Could you check a few things on this model? Use its own coordinates, in mm. A direction names the side the tool comes from. Round coordinates to 2 decimals unless told otherwise and drop trailing zeros. Order: outer loops, then holes, each group sorted by start corner. A loop starts at its lowest first (then second) coordinate and runs counter-clockwise, first axis right, second up.
```python
from build123d import *

# Parameters (mm, degrees)
RESSALTO_EXTRUS_O2_DEPTH      = 30
RESSALTO_EXTRUS_O3_START      = 3
RESSALTO_EXTRUS_O3_DEPTH      = 3
RESSALTO_EXTRUS_O4_DEPTH      = 3
RESSALTO_EXTRUS_O4_DEPTH_BACK = 10
CORTE_EXTRUS_O1_DEPTH         = 10
CORTE_EXTRUS_O2_REACH         = 83.702
FILETE1_START                 = -19.773073923
FILETE1_DEPTH                 = 36.75
FILETE1_START_2               = -13.40159992
FILETE1_2_DEPTH               = 59
ESBO_O10_R                    = 1.5
CORTE_EXTRUS_O3_DEPTH         = 10
CORTE_EXTRUS_O4_DEPTH         = 10
FILETE2_R                     = 2
ESBO_O13_R                    = 1.5
CORTE_EXTRUS_O5_DEPTH         = 16


with BuildPart() as part:
    # Esboço2 → Ressalto-extrusão2 (new body)
    with BuildSketch(Plane(origin=(0, 0, 0), x_dir=(0, 0, -1), z_dir=(1, 0, 0))):
        with BuildLine():
            Line((2.90159992, -0.062465938), (-35.09840008, -0.062465938))
            Line((-35.09840008, -0.062465938), (-39.886084903, -0.062465938))
            ThreePointArc((-39.886084903, -0.062465938), (-45.202180234, 1.467638524), (-48.891439328, 5.589707975))
            ThreePointArc((-48.891439328, 5.589707975), (-52.096536948, 9.772081499), (-56.69840008, 12.338743681))
            ThreePointArc((-56.69840008, 12.338743681), (-59.373224015, 11.895603401), (-60.59840008, 9.476926077))
            Line((-60.59840008, 9.476926077), (-60.59840008, 20.976926077))
            ThreePointArc((-60.59840008, 20.976926077), (-59.719720424, 23.09824642), (-57.59840008, 23.976926077))
            Line((-57.59840008, 23.976926077), (25.40159992, 23.976926077))
            ThreePointArc((25.40159992, 23.976926077), (27.522920263, 23.09824642), (28.40159992, 20.976926077))
            Line((28.40159992, 20.976926077), (28.40159992, 9.476926077))
            ThreePointArc((28.40159992, 9.476926077), (27.176423855, 11.895603401), (24.50159992, 12.338743681))
            ThreePointArc((24.50159992, 12.338743681), (19.899736788, 9.772081499), (16.694639168, 5.589707975))
            ThreePointArc((16.694639168, 5.589707975), (13.005380073, 1.467638524), (7.689284743, -0.062465938))
            Line((7.689284743, -0.062465938), (2.90159992, -0.062465938))
        make_face()
    extrude(amount=RESSALTO_EXTRUS_O2_DEPTH)

    # Esboço3 → Ressalto-extrusão3 (add)
    with BuildSketch(Plane.ZY.offset(RESSALTO_EXTRUS_O3_START)):
        with BuildLine():
            Line((60.59840008, 15.226926077), (60.59840008, 20.976926077))
            ThreePointArc((60.59840008, 20.976926077), (59.719720424, 23.09824642), (57.59840008, 23.976926077))
            Line((57.59840008, 23.976926077), (16.09840008, 23.976926077))
            Line((16.09840008, 23.976926077), (-25.40159992, 23.976926077))
            ThreePointArc((-25.40159992, 23.976926077), (-27.522920263, 23.09824642), (-28.40159992, 20.976926077))
            Line((-28.40159992, 20.976926077), (-28.40159992, 15.226926077))
            Line((-28.40159992, 15.226926077), (-28.40159992, -16.773073923))
            ThreePointArc((-28.40159992, -16.773073923), (-27.522920263, -18.894394267), (-25.40159992, -19.773073923))
            Line((-25.40159992, -19.773073923), (57.59840008, -19.773073923))
            ThreePointArc((57.59840008, -19.773073923), (59.719720424, -18.894394267), (60.59840008, -16.773073923))
            Line((60.59840008, -16.773073923), (60.59840008, 15.226926077))
        make_face()
    extrude(amount=-RESSALTO_EXTRUS_O3_DEPTH)

    # Esboço4 → Ressalto-extrusão4 (add, two sides: drawn at the far end of the back side and taken through both)
    with BuildSketch(Plane(origin=(30, 0, 0), x_dir=(0, 0, -1), z_dir=(1, 0, 0)).offset(-RESSALTO_EXTRUS_O4_DEPTH_BACK)):
        with BuildLine():
            Line((-16.09840008, 23.976926077), (25.40159992, 23.976926077))
            ThreePointArc((25.40159992, 23.976926077), (27.522920263, 23.09824642), (28.40159992, 20.976926077))
            Line((28.40159992, 20.976926077), (28.40159992, 15.226926077))
            Line((28.40159992, 15.226926077), (28.40159992, -16.773073923))
            ThreePointArc((28.40159992, -16.773073923), (27.522920263, -18.894394267), (25.40159992, -19.773073923))
            Line((25.40159992, -19.773073923), (-57.59840008, -19.773073923))
            ThreePointArc((-57.59840008, -19.773073923), (-59.719720424, -18.894394267), (-60.59840008, -16.773073923))
            Line((-60.59840008, -16.773073923), (-60.59840008, 15.226926077))
            Line((-60.59840008, 15.226926077), (-60.59840008, 20.976926077))
            ThreePointArc((-60.59840008, 20.976926077), (-59.719720424, 23.09824642), (-57.59840008, 23.976926077))
            Line((-57.59840008, 23.976926077), (-16.09840008, 23.976926077))
        make_face()
    extrude(amount=RESSALTO_EXTRUS_O4_DEPTH + RESSALTO_EXTRUS_O4_DEPTH_BACK)

    # Esboço8 → Corte-extrusão1 (cut)
    with BuildSketch(Plane(origin=(33, 0, 0), x_dir=(0, 0, -1), z_dir=(1, 0, 0))):
        with BuildLine():
            Line((-43.59840008, -2.773073923), (11.40159992, -2.773073923))
            ThreePointArc((11.40159992, -2.773073923), (12.815813482, -3.358860361), (13.40159992, -4.773073923))
            Line((13.40159992, -4.773073923), (13.40159992, -10.773073923))
            ThreePointArc((13.40159992, -10.773073923), (12.815813482, -12.187287486), (11.40159992, -12.773073923))
            Line((11.40159992, -12.773073923), (-43.59840008, -12.773073923))
            ThreePointArc((-43.59840008, -12.773073923), (-45.012613643, -12.187287486), (-45.59840008, -10.773073923))
            Line((-45.59840008, -10.773073923), (-45.59840008, -4.773073923))
            ThreePointArc((-45.59840008, -4.773073923), (-45.012613643, -3.358860361), (-43.59840008, -2.773073923))
        make_face()
        with BuildLine():
            Line((-43.59840008, 6.976926077), (11.40159992, 6.976926077))
            ThreePointArc((11.40159992, 6.976926077), (12.815813482, 7.562712514), (13.40159992, 8.976926077))
            Line((13.40159992, 8.976926077), (13.40159992, 14.976926077))
            ThreePointArc((13.40159992, 14.976926077), (12.815813482, 16.391139639), (11.40159992, 16.976926077))
            Line((11.40159992, 16.976926077), (-43.59840008, 16.976926077))
            ThreePointArc((-43.59840008, 16.976926077), (-45.012613643, 16.391139639), (-45.59840008, 14.976926077))
            Line((-45.59840008, 14.976926077), (-45.59840008, 8.976926077))
            ThreePointArc((-45.59840008, 8.976926077), (-45.012613643, 7.562712514), (-43.59840008, 6.976926077))
        make_face()
    extrude(amount=-CORTE_EXTRUS_O1_DEPTH, mode=Mode.SUBTRACT)

    # Corte-extrusão2: up to this face of the body (flat: up to its plane)
    corte_extrus_o2_end = Plane(part.part.faces().sort_by_distance((28, 16.976926077, 16.09840008))[0])
    # Esboço9 → Corte-extrusão2 (cut, up to the picked face)
    with BuildSketch(Plane(origin=(0, -19.773073923, 0), x_dir=(-1, 0, 0), z_dir=(0, -1, 0)), mode=Mode.PRIVATE) as corte_extrus_o2_sk1:
        with BuildLine():
            Line((-25, 13.40159992), (-28, 13.40159992))
            ThreePointArc((-28, 13.40159992), (-29.414213562, 12.815813482), (-30, 11.40159992))
            Line((-30, 11.40159992), (-30, -43.59840008))
            ThreePointArc((-30, -43.59840008), (-29.414213562, -45.012613643), (-28, -45.59840008))
            Line((-28, -45.59840008), (-25, -45.59840008))
            ThreePointArc((-25, -45.59840008), (-23.585786438, -45.012613643), (-23, -43.59840008))
            Line((-23, -43.59840008), (-23, 11.40159992))
            ThreePointArc((-23, 11.40159992), (-23.585786438, 12.815813482), (-25, 13.40159992))
        make_face()
    corte_extrus_o2_tool1 = split(extrude(corte_extrus_o2_sk1.sketch, amount=-CORTE_EXTRUS_O2_REACH, mode=Mode.PRIVATE), bisect_by=corte_extrus_o2_end, keep=Keep.BOTH, mode=Mode.PRIVATE)
    add(corte_extrus_o2_tool1.solids().sort_by(Axis((26.5, -19.773074, 16.0984), (0, 1, 0)))[0], mode=Mode.SUBTRACT)

    # Filete1: read off the stored shape, not the designer's step
    # Filete1 outline → Filete1 (add)
    with BuildSketch(Plane(origin=(0, 0, 0), x_dir=(1, 0, 0), z_dir=(0, 1, 0)).offset(FILETE1_START)):
        with BuildLine():
            ThreePointArc((25, -45.59840008), (23.585786437, -45.012613642), (23, -43.59840008))
            Line((23, -43.59840008), (23, -45.59840008))
            Line((23, -45.59840008), (25, -45.59840008))
        make_face()
        with BuildLine():
            ThreePointArc((23, 11.40159992), (23.585786438, 12.815813482), (25, 13.40159992))
            Line((25, 13.40159992), (23, 13.40159992))
            Line((23, 13.40159992), (23, 11.40159992))
        make_face()
    extrude(amount=FILETE1_DEPTH)

    # Filete1 2 outline → Filete1 2 (add)
    with BuildSketch(Plane.XY.offset(FILETE1_START_2)):
        with BuildLine():
            ThreePointArc((23, 14.976926077), (23.585786438, 16.391139639), (25, 16.976926077))
            Line((25, 16.976926077), (23, 16.976926077))
            Line((23, 16.976926077), (23, 14.976926077))
        make_face()
    extrude(amount=FILETE1_2_DEPTH)

    # Esboço10 → Corte-extrusão3 (cut)
    with BuildSketch(Plane(origin=(0, 0, 0), x_dir=(0, 0, -1), z_dir=(1, 0, 0))):
        with Locations((-55.59840008, 6.338743681)):
            Circle(ESBO_O10_R)
        with Locations((23.40159992, 6.338743681)):
            Circle(ESBO_O10_R)
        with Locations((-16.09840008, -8.562465938)):
            Circle(ESBO_O10_R)
    extrude(amount=-CORTE_EXTRUS_O3_DEPTH, mode=Mode.SUBTRACT)

    # Esboço12 → Corte-extrusão4 (cut)
    with BuildSketch(Plane(origin=(0, 0, 0), x_dir=(0, 0, -1), z_dir=(1, 0, 0))):
        with BuildLine():
            Line((-31.59840008, -2.862465938), (-25.59840008, -2.862465938))
            ThreePointArc((-25.59840008, -2.862465938), (-24.184186518, -3.448252375), (-23.59840008, -4.862465938))
            Line((-23.59840008, -4.862465938), (-23.59840008, -14.773073923))
            ThreePointArc((-23.59840008, -14.773073923), (-24.184186518, -16.187287486), (-25.59840008, -16.773073923))
            Line((-25.59840008, -16.773073923), (-31.59840008, -16.773073923))
            ThreePointArc((-31.59840008, -16.773073923), (-33.012613643, -16.187287486), (-33.59840008, -14.773073923))
            Line((-33.59840008, -14.773073923), (-33.59840008, -4.862465938))
            ThreePointArc((-33.59840008, -4.862465938), (-33.012613643, -3.448252375), (-31.59840008, -2.862465938))
        make_face()
        with BuildLine():
            Line((-6.59840008, -2.862465938), (-0.59840008, -2.862465938))
            ThreePointArc((-0.59840008, -2.862465938), (0.815813482, -3.448252375), (1.40159992, -4.862465938))
            Line((1.40159992, -4.862465938), (1.40159992, -14.773073923))
            ThreePointArc((1.40159992, -14.773073923), (0.815813482, -16.187287486), (-0.59840008, -16.773073923))
            Line((-0.59840008, -16.773073923), (-6.59840008, -16.773073923))
            ThreePointArc((-6.59840008, -16.773073923), (-8.012613643, -16.187287486), (-8.59840008, -14.773073923))
            Line((-8.59840008, -14.773073923), (-8.59840008, -4.862465938))
            ThreePointArc((-8.59840008, -4.862465938), (-8.012613643, -3.448252375), (-6.59840008, -2.862465938))
        make_face()
    extrude(amount=-CORTE_EXTRUS_O4_DEPTH, mode=Mode.SUBTRACT)

    # Filete2
    filete2_edges = [part.edges().sort_by_distance(p)[0] for p in [
        (-3, 2.101926077, 60.59840008),
        (-3, 23.09824642, 59.719720424),
        (-3, 23.976926077, 16.09840008),
        (-3, 23.09824642, -27.522920263),
        (-3, 2.101926077, -28.40159992),
        (-3, -18.894394267, -27.522920263),
        (-3, -19.773073923, 16.09840008),
        (-3, -18.894394267, 59.719720424),
    ]]
    fillet(filete2_edges, radius=FILETE2_R)

    # Esboço13 → Corte-extrusão5 (cut)
    with BuildSketch(Plane.ZY.offset(3)):
        with Locations((27.44840008, 3.976926077)):
            Circle(ESBO_O13_R)
        with Locations((4.74840008, 3.976926077)):
            Circle(ESBO_O13_R)
    extrude(amount=-CORTE_EXTRUS_O5_DEPTH, mode=Mode.SUBTRACT)


solid = part.part
```
Q1. For faces 4 (the cylindrical face through (9.86, 9.821, -19.956)), 5 (the cylindrical face through (31.09, 7.58, 45.03)), 6 (the cylindrical face through (-1.479, 6.789, 54.168)), which set-ups out of +Z, -Z, +X, -X, +Y, -Y let a thin tool reach every point of the face, with its end or its side?
Q2. Imagine slicing it at B-B, the plane x = 17. Please give me the cut outline in (y, z).
Q3. For P1, Ø1.8, axis at y = 3.98, z = 4.75, coming from the -X side; P2, Ø2.5, axis at y = -8.56, z = 16.1, coming from the -X side; P3, Ø1, axis at x = 8, z = -8.5, coming from the -Y side; P4, Ø4, axis at x = 17, y = -9.5, coming from the +Z side, each with a flat end and sliding along its axis, tell me the tip position at first contact or that it passes through.
Q4. Imagine slicing it at D-D, the plane z = 28. State how many separate pieces and enclosed holes the cut face has, then the cut area to 3 significant figures.
Q5. We'd pull the mould along Z, two halves only. Please class faces 1 (the flat face through (-3, 2, 16)), 2 (the flat face through (13, 4, 27)), 3 (the cylindrical face through (15.762, 23.075, 59.743)): released by +Z, released by -Z, zero draft, split by the parting line, or undercut.
Q6. Imagine slicing it at C-C, the plane y = 11. Please give me the cut outline in (x, z).
Q7. Imagine slicing it at A-A, the plane z = -6.5. Please give me the cut outline in (x, y), then the cut area to 3 significant figures.
Q8. I need wall thicknesses on L1, parallel to X at y = -16, z = 4; L2, parallel to Y at x = 31.5, z = -9; L3, parallel to X at y = -6, z = -6.5. Which ranges of each line are inside material? Lowest first, please.
Filled in:
1. face 4: -Y
1. face 5: +X
1. face 6: -X
2. outline: (-0.06, -7.69) arc R10 ccw to (5.59, -16.69) arc R13 cw to (12.34, -24.5) arc R3 cw to (9.48, -28.4) - (20.98, -28.4) arc R3 ccw to (23.98, -25.4) - (23.98, 57.6) arc R3 ccw to (20.98, 60.6) - (9.48, 60.6) arc R3 cw to (12.34, 56.7) arc R13 cw to (5.59, 48.89) arc R10 ccw to (-0.06, 39.89) - close
3. P1: stops at x = 13
3. P2: stops at x = 20
3. P3: stops at y = -0.06
3. P4: passes through
4. separate pieces: 4
4. enclosed holes: 0
4. area: 776 mm2
5. face 1: zero draft
5. face 2: undercut
5. face 3: released by +Z
6. outline: (-3, -26.4) arc R2 ccw to (-1, -28.4) - (33, -28.4) - (33, -13.4) - (25, -13.4) arc R2 cw to (23, -11.4) - (23, 43.6) arc R2 cw to (25, 45.6) - (33, 45.6) - (33, 60.6) - (-1, 60.6) arc R2 ccw to (-3, 58.6) - close; hole (0, -27.99) - (20, -27.99) - (20, -21.57) - (0, -21.57) - close; hole (0, 53.77) - (20, 53.77) - (20, 60.18) - (0, 60.18) - close
7. outline: (-3, -17.77) arc R2 ccw to (-1, -19.77) - (0, -19.77) - (0, -0.06) - (20, -0.06) - (20, -19.77) - (23, -19.77) - (23, 14.98) arc R2 cw to (25, 16.98) - (33, 16.98) - (33, 23.98) - (-1, 23.98) arc R2 ccw to (-3, 21.98) - close; (30, -19.77) - (33, -19.77) - (33, -12.77) - (30, -12.77) - close; (30, -2.77) - (33, -2.77) - (33, 6.98) - (30, 6.98) - close
7. area: 863 mm2
8. L1: x = 20 to 23, 30 to 33
8. L2: y = -19.77 to -12.77, -2.77 to 6.98, 16.98 to 23.98
8. L3: x = -3 to 0, 20 to 23
